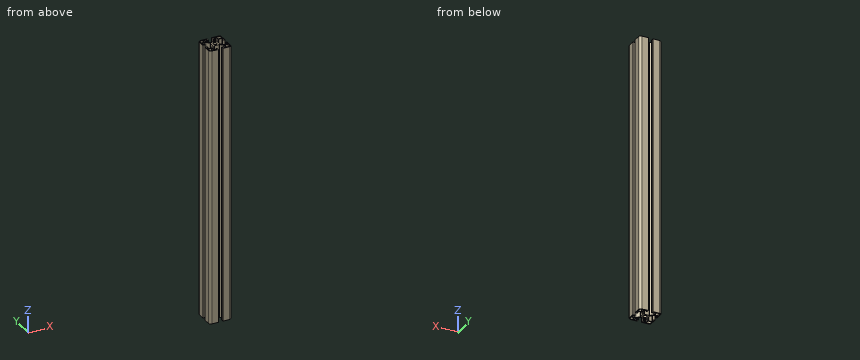
```python
from build123d import *

# Parameters (mm, degrees)
SKETCH1_R           = 3.4
BOSS_EXTRUDE1_DEPTH = 500


with BuildPart() as part:
    # Sketch1 → Boss-Extrude1 (new body)
    with BuildSketch(Plane.XY):
        with BuildLine():
            Line((-20, 4.1), (-20, 15.5))
            ThreePointArc((-20, 15.5), (-18.681980515, 18.681980515), (-15.5, 20))
            Line((-15.5, 20), (-4.1, 20))
            Line((-4.1, 20), (-4.1, 15.8))
            ThreePointArc((-4.1, 15.8), (-4.187867966, 15.587867966), (-4.4, 15.5))
            Line((-4.4, 15.5), (-6.1, 15.5))
            ThreePointArc((-6.1, 15.5), (-6.312132034, 15.587867966), (-6.4, 15.8))
            Line((-6.4, 15.8), (-6.4, 17.5))
            ThreePointArc((-6.4, 17.5), (-6.692893219, 18.207106781), (-7.4, 18.5))
            Line((-7.4, 18.5), (-9.25, 18.5))
            ThreePointArc((-9.25, 18.5), (-9.957106781, 18.207106781), (-10.25, 17.5))
            Line((-10.25, 17.5), (-10.25, 12.492640687))
            ThreePointArc((-10.25, 12.492640687), (-10.097759065, 11.727273822), (-9.664213562, 11.078427125))
            Line((-9.664213562, 11.078427125), (-5.171572875, 6.585786438))
            ThreePointArc((-5.171572875, 6.585786438), (-4.522726178, 6.152240935), (-3.757359313, 6))
            Line((-3.757359313, 6), (3.757359313, 6))
            ThreePointArc((3.757359313, 6), (4.522726178, 6.152240935), (5.171572875, 6.585786438))
            Line((5.171572875, 6.585786438), (9.664213562, 11.078427125))
            ThreePointArc((9.664213562, 11.078427125), (10.097759065, 11.727273822), (10.25, 12.492640687))
            Line((10.25, 12.492640687), (10.25, 17.5))
            ThreePointArc((10.25, 17.5), (9.957106781, 18.207106781), (9.25, 18.5))
            Line((9.25, 18.5), (7.4, 18.5))
            ThreePointArc((7.4, 18.5), (6.692893219, 18.207106781), (6.4, 17.5))
            Line((6.4, 17.5), (6.4, 15.8))
            ThreePointArc((6.4, 15.8), (6.312132034, 15.587867966), (6.1, 15.5))
            Line((6.1, 15.5), (4.4, 15.5))
            ThreePointArc((4.4, 15.5), (4.187867966, 15.587867966), (4.1, 15.8))
            Line((4.1, 15.8), (4.1, 20))
            Line((4.1, 20), (15.5, 20))
            ThreePointArc((15.5, 20), (18.681980515, 18.681980515), (20, 15.5))
            Line((20, 15.5), (20, 4.1))
            Line((20, 4.1), (15.8, 4.1))
            ThreePointArc((15.8, 4.1), (15.587867966, 4.187867966), (15.5, 4.4))
            Line((15.5, 4.4), (15.5, 6.1))
            ThreePointArc((15.5, 6.1), (15.587867966, 6.312132034), (15.8, 6.4))
            Line((15.8, 6.4), (17.5, 6.4))
            ThreePointArc((17.5, 6.4), (18.207106781, 6.692893219), (18.5, 7.4))
            Line((18.5, 7.4), (18.5, 9.25))
            ThreePointArc((18.5, 9.25), (18.207106781, 9.957106781), (17.5, 10.25))
            Line((17.5, 10.25), (12.492640687, 10.25))
            ThreePointArc((12.492640687, 10.25), (11.727273822, 10.097759065), (11.078427125, 9.664213562))
            Line((11.078427125, 9.664213562), (6.585786438, 5.171572875))
            ThreePointArc((6.585786438, 5.171572875), (6.152240935, 4.522726178), (6, 3.757359313))
            Line((6, 3.757359313), (6, -3.757359313))
            ThreePointArc((6, -3.757359313), (6.152240935, -4.522726178), (6.585786438, -5.171572875))
            Line((6.585786438, -5.171572875), (11.078427125, -9.664213562))
            ThreePointArc((11.078427125, -9.664213562), (11.727273822, -10.097759065), (12.492640687, -10.25))
            Line((12.492640687, -10.25), (17.5, -10.25))
            ThreePointArc((17.5, -10.25), (18.207106781, -9.957106781), (18.5, -9.25))
            Line((18.5, -9.25), (18.5, -7.4))
            ThreePointArc((18.5, -7.4), (18.207106781, -6.692893219), (17.5, -6.4))
            Line((17.5, -6.4), (15.8, -6.4))
            ThreePointArc((15.8, -6.4), (15.587867966, -6.312132034), (15.5, -6.1))
            Line((15.5, -6.1), (15.5, -4.4))
            ThreePointArc((15.5, -4.4), (15.587867966, -4.187867966), (15.8, -4.1))
            Line((15.8, -4.1), (20, -4.1))
            Line((20, -4.1), (20, -15.5))
            ThreePointArc((20, -15.5), (18.681980515, -18.681980515), (15.5, -20))
            Line((15.5, -20), (4.1, -20))
            Line((4.1, -20), (4.1, -15.8))
            ThreePointArc((4.1, -15.8), (4.187867966, -15.587867966), (4.4, -15.5))
            Line((4.4, -15.5), (6.1, -15.5))
            ThreePointArc((6.1, -15.5), (6.312132034, -15.587867966), (6.4, -15.8))
            Line((6.4, -15.8), (6.4, -17.5))
            ThreePointArc((6.4, -17.5), (6.692893219, -18.207106781), (7.4, -18.5))
            Line((7.4, -18.5), (9.25, -18.5))
            ThreePointArc((9.25, -18.5), (9.957106781, -18.207106781), (10.25, -17.5))
            Line((10.25, -17.5), (10.25, -12.492640687))
            ThreePointArc((10.25, -12.492640687), (10.097759065, -11.727273822), (9.664213562, -11.078427125))
            Line((9.664213562, -11.078427125), (5.171572875, -6.585786438))
            ThreePointArc((5.171572875, -6.585786438), (4.522726178, -6.152240935), (3.757359313, -6))
            Line((3.757359313, -6), (-3.757359313, -6))
            ThreePointArc((-3.757359313, -6), (-4.522726178, -6.152240935), (-5.171572875, -6.585786438))
            Line((-5.171572875, -6.585786438), (-9.664213562, -11.078427125))
            ThreePointArc((-9.664213562, -11.078427125), (-10.097759065, -11.727273822), (-10.25, -12.492640687))
            Line((-10.25, -12.492640687), (-10.25, -17.5))
            ThreePointArc((-10.25, -17.5), (-9.957106781, -18.207106781), (-9.25, -18.5))
            Line((-9.25, -18.5), (-7.4, -18.5))
            ThreePointArc((-7.4, -18.5), (-6.692893219, -18.207106781), (-6.4, -17.5))
            Line((-6.4, -17.5), (-6.4, -15.8))
            ThreePointArc((-6.4, -15.8), (-6.312132034, -15.587867966), (-6.1, -15.5))
            Line((-6.1, -15.5), (-4.4, -15.5))
            ThreePointArc((-4.4, -15.5), (-4.187867966, -15.587867966), (-4.1, -15.8))
            Line((-4.1, -15.8), (-4.1, -20))
            Line((-4.1, -20), (-15.5, -20))
            ThreePointArc((-15.5, -20), (-18.681980515, -18.681980515), (-20, -15.5))
            Line((-20, -15.5), (-20, -4.1))
            Line((-20, -4.1), (-15.8, -4.1))
            ThreePointArc((-15.8, -4.1), (-15.587867966, -4.187867966), (-15.5, -4.4))
            Line((-15.5, -4.4), (-15.5, -6.1))
            ThreePointArc((-15.5, -6.1), (-15.587867966, -6.312132034), (-15.8, -6.4))
            Line((-15.8, -6.4), (-17.5, -6.4))
            ThreePointArc((-17.5, -6.4), (-18.207106781, -6.692893219), (-18.5, -7.4))
            Line((-18.5, -7.4), (-18.5, -9.25))
            ThreePointArc((-18.5, -9.25), (-18.207106781, -9.957106781), (-17.5, -10.25))
            Line((-17.5, -10.25), (-12.492640687, -10.25))
            ThreePointArc((-12.492640687, -10.25), (-11.727273822, -10.097759065), (-11.078427125, -9.664213562))
            Line((-11.078427125, -9.664213562), (-6.585786438, -5.171572875))
            ThreePointArc((-6.585786438, -5.171572875), (-6.152240935, -4.522726178), (-6, -3.757359313))
            Line((-6, -3.757359313), (-6, 3.757359313))
            ThreePointArc((-6, 3.757359313), (-6.152240935, 4.522726178), (-6.585786438, 5.171572875))
            Line((-6.585786438, 5.171572875), (-11.078427125, 9.664213562))
            ThreePointArc((-11.078427125, 9.664213562), (-11.727273822, 10.097759065), (-12.492640687, 10.25))
            Line((-12.492640687, 10.25), (-17.5, 10.25))
            ThreePointArc((-17.5, 10.25), (-18.207106781, 9.957106781), (-18.5, 9.25))
            Line((-18.5, 9.25), (-18.5, 7.4))
            ThreePointArc((-18.5, 7.4), (-18.207106781, 6.692893219), (-17.5, 6.4))
            Line((-17.5, 6.4), (-15.8, 6.4))
            ThreePointArc((-15.8, 6.4), (-15.587867966, 6.312132034), (-15.5, 6.1))
            Line((-15.5, 6.1), (-15.5, 4.4))
            ThreePointArc((-15.5, 4.4), (-15.587867966, 4.187867966), (-15.8, 4.1))
            Line((-15.8, 4.1), (-20, 4.1))
        make_face()
        Circle(SKETCH1_R, mode=Mode.SUBTRACT)
        with BuildLine():
            Line((18.7, 12.55), (18.7, 15.5))
            ThreePointArc((18.7, 15.5), (17.7627417, 17.7627417), (15.5, 18.7))
            Line((15.5, 18.7), (12.55, 18.7))
            ThreePointArc((12.55, 18.7), (11.842893219, 18.407106781), (11.55, 17.7))
            Line((11.55, 17.7), (11.55, 12.55))
            ThreePointArc((11.55, 12.55), (11.842893219, 11.842893219), (12.55, 11.55))
            Line((12.55, 11.55), (17.7, 11.55))
            ThreePointArc((17.7, 11.55), (18.407106781, 11.842893219), (18.7, 12.55))
        make_face(mode=Mode.SUBTRACT)
        with BuildLine():
            Line((-18.7, -12.55), (-18.7, -15.5))
            ThreePointArc((-18.7, -15.5), (-17.7627417, -17.7627417), (-15.5, -18.7))
            Line((-15.5, -18.7), (-12.55, -18.7))
            ThreePointArc((-12.55, -18.7), (-11.842893219, -18.407106781), (-11.55, -17.7))
            Line((-11.55, -17.7), (-11.55, -12.55))
            ThreePointArc((-11.55, -12.55), (-11.842893219, -11.842893219), (-12.55, -11.55))
            Line((-12.55, -11.55), (-17.7, -11.55))
            ThreePointArc((-17.7, -11.55), (-18.407106781, -11.842893219), (-18.7, -12.55))
        make_face(mode=Mode.SUBTRACT)
        with BuildLine():
            Line((-12.55, 18.7), (-15.5, 18.7))
            ThreePointArc((-15.5, 18.7), (-17.7627417, 17.7627417), (-18.7, 15.5))
            Line((-18.7, 15.5), (-18.7, 12.55))
            ThreePointArc((-18.7, 12.55), (-18.407106781, 11.842893219), (-17.7, 11.55))
            Line((-17.7, 11.55), (-12.55, 11.55))
            ThreePointArc((-12.55, 11.55), (-11.842893219, 11.842893219), (-11.55, 12.55))
            Line((-11.55, 12.55), (-11.55, 17.7))
            ThreePointArc((-11.55, 17.7), (-11.842893219, 18.407106781), (-12.55, 18.7))
        make_face(mode=Mode.SUBTRACT)
        with BuildLine():
            Line((12.55, -18.7), (15.5, -18.7))
            ThreePointArc((15.5, -18.7), (17.7627417, -17.7627417), (18.7, -15.5))
            Line((18.7, -15.5), (18.7, -12.55))
            ThreePointArc((18.7, -12.55), (18.407106781, -11.842893219), (17.7, -11.55))
            Line((17.7, -11.55), (12.55, -11.55))
            ThreePointArc((12.55, -11.55), (11.842893219, -11.842893219), (11.55, -12.55))
            Line((11.55, -12.55), (11.55, -17.7))
            ThreePointArc((11.55, -17.7), (11.842893219, -18.407106781), (12.55, -18.7))
        make_face(mode=Mode.SUBTRACT)
    extrude(amount=BOSS_EXTRUDE1_DEPTH)


solid = part.part
```
The listing builds one solid part. Answer for the finished solid, in the listing's coordinates (mm). Coordinates: 2 decimals unless noted, no trailing zeros. Answer as a JSON object with one key per item and string values. Group by question number.
1. Section A-A on z = 165.5 is taken. State how many separate pieces and enclosed holes the cut face has, then the cut area to 3 significant figures.
2. Flat-ended cylindrical pins translate along their axes: P1, Ø3.5, axis at x = 17.5, z = 334, coming from the +Y side; P2, Ø4.5, axis at x = -18.5, z = 179.5, coming from the +Y side; P3, Ø4, axis at x = -2, z = 200, coming from the +Y side. Find the tip coordinate at first contact, or state that the pin passes through.
3. Straight lines are drawn through the part: line 1 (Y direction, x = -14, z = 199); line 2 (Y direction, x = -4.5, z = 102). For each, find the intervals that lie inside material, in ascending order.
Values follow:
{
 "1": {"separate pieces": "1", "enclosed holes": "5", "area": "467 mm2"},
 "2": {"P1": "y = 19.99", "P2": "y = 19.94", "P3": "y = 6.01"},
 "3": {"line 1": "-20 to -18.7, -11.55 to -10.25, 10.25 to 11.55, 18.7 to 20", "line 2": "-20 to -15.5, -6.14 to 6.14, 15.5 to 20"}
}
